from build123d import *

# Parameters (mm, degrees)
SKETCH1_W                = 15.875
SKETCH1_H                = 15.875
BOSS_EXTRUDE1_DEPTH      = 31.75
BOSS_EXTRUDE3_DEPTH      = 3.175
BOSS_EXTRUDE3_DEPTH_BACK = 3.175
SKETCH4_R                = 1.190625
CUT_EXTRUDE1_DEPTH       = 16.875
SKETCH8_R                = 1.5875
CUT_EXTRUDE3_DEPTH       = 7.9375
SKETCH7_R                = 1.5875
CUT_EXTRUDE4_DEPTH       = 7.9375
SKETCH10_W               = 9.525
SKETCH10_H               = 4.7625
CUT_EXTRUDE5_DEPTH       = 32.75
CUT_EXTRUDE6_DEPTH       = 12.1125


with BuildPart() as part:
    # Sketch1 → Boss-Extrude1 (new body)
    with BuildSketch(Plane.XY):
        Rectangle(SKETCH1_W, SKETCH1_H)
    extrude(amount=BOSS_EXTRUDE1_DEPTH)

    # Sketch3 → Boss-Extrude3 (add, two sides)
    with BuildSketch(Plane(origin=(0, 0, 0), x_dir=(1, 0, 0), z_dir=(0, 1, 0))) as boss_extrude3_sk:
        with BuildLine():
            Line((-7.9375, 0), (7.9375, 0))
            ThreePointArc((7.9375, 0), (0, 7.9375), (-7.9375, 0))
        make_face()
    extrude(amount=BOSS_EXTRUDE3_DEPTH)
    extrude(boss_extrude3_sk.sketch, amount=-BOSS_EXTRUDE3_DEPTH_BACK)

    # Sketch4 → Cut-Extrude1 (cut, through all)
    with BuildSketch(Plane(origin=(7.9375, 0, 0), x_dir=(0, 0, -1), z_dir=(1, 0, 0))):
        with Locations((-15.875, 0)):
            Circle(SKETCH4_R)
    extrude(amount=-CUT_EXTRUDE1_DEPTH, mode=Mode.SUBTRACT)

    # Sketch8 → Cut-Extrude3 (cut)
    with BuildSketch(Plane(origin=(4.72140587, 0, -6.380613831), x_dir=(-0.803856861, 0, -0.594822787), z_dir=(0.594822787, 0, -0.803856861))):
        Circle(SKETCH8_R)
    extrude(amount=-CUT_EXTRUDE3_DEPTH, mode=Mode.SUBTRACT)

    # Sketch7 → Cut-Extrude4 (cut)
    with BuildSketch(Plane(origin=(-6.380613831, 0, -4.72140587), x_dir=(0.594822787, 0, -0.803856861), z_dir=(0.803856861, 0, 0.594822787))):
        Circle(SKETCH7_R)
    extrude(amount=CUT_EXTRUDE4_DEPTH, mode=Mode.SUBTRACT)

    # Sketch10 → Cut-Extrude5 (cut, through all)
    with BuildSketch(Plane(origin=(0, 0, 0), x_dir=(-1, 0, 0), z_dir=(0, 0, -1))):
        with Locations((0, 5.55625)):
            Rectangle(SKETCH10_W, SKETCH10_H)
        with Locations((0, -5.55625)):
            Rectangle(SKETCH10_W, SKETCH10_H)
    extrude(amount=-CUT_EXTRUDE5_DEPTH, mode=Mode.SUBTRACT)

    # Sketch12 → Cut-Extrude6 (cut, through all)
    with BuildSketch(Plane(origin=(0, 3.175, 0), x_dir=(1, 0, 0), z_dir=(0, 1, 0))):
        with BuildLine():
            Line((-3.175, -25.4), (-3.175, -6.35))
            ThreePointArc((-3.175, -6.35), (0, -3.175), (3.175, -6.35))
            Line((3.175, -6.35), (3.175, -25.4))
            ThreePointArc((3.175, -25.4), (0, -28.575), (-3.175, -25.4))
        make_face()
    extrude(amount=-CUT_EXTRUDE6_DEPTH, mode=Mode.SUBTRACT)


solid = part.part
Input: part model. Units: mm. Frame: model coordinates. A direction names the side the tool comes from. Give positions to 0.01 mm unless a question says otherwise; leave off trailing zeros. Order: outer loops, then holes, each group sorted by start corner. A loop starts at its lowest first (then second) coordinate and runs counter-clockwise, first axis right, second up. Notation, with made-up numbers: (82.5, 89.5) - (90.5, 89.5) arc R26 cw to (90.5, 113.5) - close; hole circle Ø1 at (-31.75, 58.5). An arc over 180 degrees is marked (long way). Answer as a JSON object with one key per item and string values. Group by question number.
Q1. Line query: probe 1 along X at (y, z) = (3, 20) (1 decimal); probe 2 along X at (y, z) = (6.75, 30.5); probe 3 along Y at (x, z) = (1.5, 1.5) (3 decimals). Output: solid intervals per line, ascending.
Q2. Cut plane A-A, the plane z = 13.5. Output: boundary loops of the cut face in (x, y) (1 decimal), then the cut area to 3 significant figures.
Q3. Cut plane C-C, the plane y = 0. Count the separate pieces of the cut face and the enclosed holes in it, then the cut area to 3 significant figures.
Q4. Cut plane D-D, the plane z = 26.5. Output: boundary loops of the cut face in (x, y) (1 decimal).
Q5. Set-up query: faces 1 (the face through (-6, 6, 0)), 2 (the face through (-4.762, 6, 16)), 3 (the face through (-0.07, 0.044, 3.176)). Return all of +Z, -Z, +X, -X, +Y, -Y with unobstructed straight access to the full face (end or side cutting, diameter ignored); none if empty.
Q6. Mould query, pull axis Z, two halves, no side actions, for faces 4 (the face through (-5.523, 0.052, 17.064)), 5 (the face through (0, 0, 31.75)), 6 (the face through (4.762, -6, 16)). Classes: pulls with the +Z half, pulls with the -Z half, needs draft (parallel to the pull), parting line crosses it, or undercut.
Q7. First-contact query: pin 1 Ø5 at (x, y) = (-6, 0.5) entering from -Z; pin 2 Ø4 at (y, z) = (6, -1) entering from -X; pin 3 Ø3.5 at (x, y) = (-6.5, 6) entering from -Z; pin 4 Ø4 at (x, y) = (2.5, -5.5) entering from -Z. Flat tips, straight axial feed; report the tip coordinate or a pass-through.
Results:
{
 "1": {"probe 1": "-7.9 to -3.2, 3.2 to 7.9", "probe 2": "-7.94 to -4.76, 4.76 to 7.94", "probe 3": "-3.175 to 3.175"},
 "2": {"outline": "(-7.9, -7.9) - (-4.8, -7.9) - (-4.8, -3.2) - (-3.2, -3.2) - (-3.2, 3.2) - (-4.8, 3.2) - (-4.8, 7.9) - (-7.9, 7.9) - close; (3.2, -3.2) - (4.8, -3.2) - (4.8, -7.9) - (7.9, -7.9) - (7.9, 7.9) - (4.8, 7.9) - (4.8, 3.2) - (3.2, 3.2) - close", "area": "121 mm^2"},
 "3": {"separate pieces": "3", "enclosed holes": "0", "area": "380 mm^2"},
 "4": {"outline": "(-7.9, -7.9) - (-4.8, -7.9) - (-4.8, -3.2) - (-3, -3.2) - (-3, 3.2) - (-4.8, 3.2) - (-4.8, 7.9) - (-7.9, 7.9) - close; (3, -3.2) - (4.8, -3.2) - (4.8, -7.9) - (7.9, -7.9) - (7.9, 7.9) - (4.8, 7.9) - (4.8, 3.2) - (3, 3.2) - close"},
 "5": {"face 1": "-Z, +X, -X, +Y", "face 2": "+Z, -Z, +Y", "face 3": "+Y, -Y"},
 "6": {"face 4": "undercut", "face 5": "pulls with the +Z half", "face 6": "needs draft"},
 "7": {"pin 1": "z = -7.12", "pin 2": "x = -7.94", "pin 3": "z = 0", "pin 4": "through"}
}
